```python
from build123d import *

# Parameters (mm, degrees)
SKETCH5_W                                         = 129.54
SKETCH5_H                                         = 88.9
BUTTON_SUPPORT_DEPTH                              = 48.768
SKETCH6_W                                         = 111.76
SKETCH6_H                                         = 60.96
SKETCH6_W_2                                       = 101.6
SKETCH6_H_2                                       = 50.8
BOSS_EXTRUDE4_DEPTH                               = 6.35
SKETCH7_W                                         = 82.55
SKETCH7_H                                         = 50.8
FORCE_SENSOR_CUTOUT_DEPTH                         = 3.81
SKETCH4_W                                         = 129.54
SKETCH4_H                                         = 40.64
BOTTOM_CUT_DEPTH                                  = 139.7
SKETCH25_W                                        = 111.76
SKETCH25_H                                        = 13.97
NEOPIXEL_LIFT_DEPTH                               = 1.778
SKETCH8_W                                         = 5.08
SKETCH8_H                                         = 6.35
HAPTIC_WIRE_HOLES_DEPTH                           = 4.318
SKETCH9_W                                         = 12.7
SKETCH9_H                                         = 12.7
FORCE_SENSOR_HOLE_DEPTH                           = 4.318
SKETCH10_R                                        = 1.0795
NEOPIXEL_HOLES_DEPTH                              = 9.906
NEOPIXEL_WIRE_SIDE_HOLES_REACH                    = 10.128
SKETCH18_W                                        = 8.89
SKETCH18_H                                        = 60.96
SKETCH19_W                                        = 12.7
SKETCH19_H                                        = 13.97
SKETCH19_W_2                                      = 17.78
NEOPIXEL_SOLDER_GAP_DEPTH                         = 5.08
BOSS_EXTRUDE6_DEPTH                               = 1.27
SKETCH11_W                                        = 88.9
SKETCH11_H                                        = 8.128
BOSS_EXTRUDE5_DEPTH                               = 10.16
CSK_FOR_8_FLAT_HEAD_MACHINE_SCREW_100_D           = 4.4958
CSK_FOR_8_FLAT_HEAD_MACHINE_SCREW_100_CSINK_D     = 8.4328
CSK_FOR_8_FLAT_HEAD_MACHINE_SCREW_100_CSINK_ANGLE = 100
SKETCH23_W                                        = 12.7
SKETCH23_H                                        = 13.97
SKETCH23_H_2                                      = 15.24
CUT_EXTRUDE1_DEPTH                                = 5.826
SKETCH24_W                                        = 6.858
SKETCH24_H                                        = 6.35
CUT_EXTRUDE2_DEPTH                                = 121.65


with BuildPart() as part:
    # Sketch5 → Button Support (new body)
    with BuildSketch(Plane(origin=(0, 5.08, 0), x_dir=(1, 0, 0), z_dir=(0, 1, 0))):
        with Locations((69.85, 60.96)):
            Rectangle(SKETCH5_W, SKETCH5_H)
    extrude(amount=BUTTON_SUPPORT_DEPTH)

    # Sketch6 → Boss-Extrude4 (add)
    with BuildSketch(Plane(origin=(0, 53.848, 0), x_dir=(1, 0, 0), z_dir=(0, 1, 0))):
        with Locations((69.85, 60.96)):
            Rectangle(SKETCH6_W, SKETCH6_H)
        with Locations((69.85, 60.96)):
            Rectangle(SKETCH6_W_2, SKETCH6_H_2, mode=Mode.SUBTRACT)
    extrude(amount=BOSS_EXTRUDE4_DEPTH)

    # Sketch7 → Force Sensor Cutout (cut)
    with BuildSketch(Plane(origin=(0, 53.848, 0), x_dir=(1, 0, 0), z_dir=(0, 1, 0))):
        with Locations((69.85, 60.96)):
            Rectangle(SKETCH7_W, SKETCH7_H)
    extrude(amount=-FORCE_SENSOR_CUTOUT_DEPTH, mode=Mode.SUBTRACT)

    # Sketch4 → Bottom Cut (cut)
    with BuildSketch(Plane.XY):
        with Locations((69.85, 25.4)):
            Rectangle(SKETCH4_W, SKETCH4_H)
    extrude(amount=-BOTTOM_CUT_DEPTH, mode=Mode.SUBTRACT)

    # Sketch25 → NeoPixel Lift (add)
    with BuildSketch(Plane(origin=(0, 53.848, 0), x_dir=(1, 0, 0), z_dir=(0, 1, 0))):
        with Locations((69.85, 98.425)):
            Rectangle(SKETCH25_W, SKETCH25_H)
        with Locations((69.85, 23.495)):
            Rectangle(SKETCH25_W, SKETCH25_H)
    extrude(amount=NEOPIXEL_LIFT_DEPTH)

    # Sketch8 → Haptic Wire Holes (cut)
    with BuildSketch(Plane(origin=(0, 50.038, 0), x_dir=(1, 0, 0), z_dir=(0, 1, 0))):
        with Locations((72.898, 67.528002358)):
            Rectangle(SKETCH8_W, SKETCH8_H)
        with Locations((98.298, 67.528002358)):
            Rectangle(SKETCH8_W, SKETCH8_H)
        with Locations((47.498, 67.528002358)):
            Rectangle(SKETCH8_W, SKETCH8_H)
    extrude(amount=-HAPTIC_WIRE_HOLES_DEPTH, mode=Mode.SUBTRACT)

    # Sketch9 → Force Sensor Hole (cut)
    with BuildSketch(Plane(origin=(0, 50.038, 0), x_dir=(1, 0, 0), z_dir=(0, 1, 0))):
        with Locations((46.355, 57.15)):
            Rectangle(SKETCH9_W, SKETCH9_H)
    extrude(amount=-FORCE_SENSOR_HOLE_DEPTH, mode=Mode.SUBTRACT)

    # Sketch10 → NeoPixel Holes (cut)
    with BuildSketch(Plane(origin=(0, 55.626, 0), x_dir=(1, 0, 0), z_dir=(0, 1, 0))):
        with Locations((108.018583302, 19.2294764)):
            Circle(SKETCH10_R)
        with Locations((82.42609372, 19.2294764)):
            Circle(SKETCH10_R)
        with Locations((56.918583394, 19.2294764)):
            Circle(SKETCH10_R)
        with Locations((31.326093812, 19.2294764)):
            Circle(SKETCH10_R)
        with Locations((31.326093812, 102.6905236)):
            Circle(SKETCH10_R)
        with Locations((56.918583394, 102.6905236)):
            Circle(SKETCH10_R)
        with Locations((82.42609372, 102.6905236)):
            Circle(SKETCH10_R)
        with Locations((108.018583302, 102.6905236)):
            Circle(SKETCH10_R)
    extrude(amount=-NEOPIXEL_HOLES_DEPTH, mode=Mode.SUBTRACT)

    # Sketch18 → Neopixel Wire Side Holes (cut, up to next)
    with BuildSketch(Plane(origin=(0, 53.848, 0), x_dir=(1, 0, 0), z_dir=(0, 1, 0)), mode=Mode.PRIVATE) as neopixel_wire_side_holes_sk1:
        with Locations((130.175, 60.96)):
            Rectangle(SKETCH18_W, SKETCH18_H)
    neopixel_wire_side_holes_tool1 = extrude(neopixel_wire_side_holes_sk1.sketch, amount=-NEOPIXEL_WIRE_SIDE_HOLES_REACH, mode=Mode.PRIVATE) & part.part
    add(neopixel_wire_side_holes_tool1.solids().sort_by_distance((130.175, 53.848, -60.96))[0], mode=Mode.SUBTRACT)
    # Sketch18 → Neopixel Wire Side Holes (cut, up to next)
    with BuildSketch(Plane(origin=(0, 53.848, 0), x_dir=(1, 0, 0), z_dir=(0, 1, 0)), mode=Mode.PRIVATE) as neopixel_wire_side_holes_sk2:
        with Locations((9.525, 60.96)):
            Rectangle(SKETCH18_W, SKETCH18_H)
    neopixel_wire_side_holes_tool2 = extrude(neopixel_wire_side_holes_sk2.sketch, amount=-NEOPIXEL_WIRE_SIDE_HOLES_REACH, mode=Mode.PRIVATE) & part.part
    add(neopixel_wire_side_holes_tool2.solids().sort_by_distance((9.525, 53.848, -60.96))[0], mode=Mode.SUBTRACT)

    # Sketch19 → NeoPixel solder gap (cut)
    with BuildSketch(Plane(origin=(0, 55.626, 0), x_dir=(1, 0, 0), z_dir=(0, 1, 0))):
        with Locations((69.85, 98.425)):
            Rectangle(SKETCH19_W, SKETCH19_H)
        with Locations((13.97, 98.425)):
            Rectangle(SKETCH19_W_2, SKETCH19_H)
        with Locations((125.73, 98.425)):
            Rectangle(SKETCH19_W_2, SKETCH19_H)
    neopixel_solder_gap = extrude(amount=-NEOPIXEL_SOLDER_GAP_DEPTH, mode=Mode.SUBTRACT)

    # Mirror1: NeoPixel solder gap across plane
    add(neopixel_solder_gap.mirror(Plane.XY.offset(-60.96)), mode=Mode.SUBTRACT)

    # Sketch20 → Boss-Extrude6 (add)
    with BuildSketch(Plane.XY.offset(-16.51)):
        Polygon((22.86, 50.546), (5.08, 50.546), (5.08, 45.786808958), (134.62, 45.786808958), (134.62, 50.546), (116.84, 50.546), (116.84, 53.848), (76.2, 53.848), (76.2, 50.546), (63.5, 50.546), (63.5, 53.848), (22.86, 53.848), align=None)
    extrude(amount=BOSS_EXTRUDE6_DEPTH)

    # Sketch11 → Boss-Extrude5 (add)
    with BuildSketch(Plane.XY.offset(-15.24)):
        with Locations((69.85, 49.784)):
            Rectangle(SKETCH11_W, SKETCH11_H)
    extrude(amount=BOSS_EXTRUDE5_DEPTH)

    # CSK for #8 Flat Head Machine Screw (100)1 (through all)
    with Locations(Plane(origin=(0, 50.546, 0), x_dir=(1, 0, 0), z_dir=(0, 1, 0))):
        with Locations((12.7, 99.06), (127, 99.06), (127, 21.59), (12.7, 21.59)):
            CounterSinkHole(CSK_FOR_8_FLAT_HEAD_MACHINE_SCREW_100_D / 2, CSK_FOR_8_FLAT_HEAD_MACHINE_SCREW_100_CSINK_D / 2, counter_sink_angle=CSK_FOR_8_FLAT_HEAD_MACHINE_SCREW_100_CSINK_ANGLE)

    # Sketch23 → Cut-Extrude1 (cut, through all)
    with BuildSketch(Plane(origin=(0, 50.546, 0), x_dir=(1, 0, 0), z_dir=(0, 1, 0))):
        with Locations((69.85, 98.425)):
            Rectangle(SKETCH23_W, SKETCH23_H)
        with Locations((69.85, 22.86)):
            Rectangle(SKETCH23_W, SKETCH23_H_2)
    extrude(amount=-CUT_EXTRUDE1_DEPTH, mode=Mode.SUBTRACT)

    # Sketch24 → Cut-Extrude2 (cut, through all)
    with BuildSketch(Plane(origin=(125.73, 0, 0), x_dir=(0, 0, -1), z_dir=(1, 0, 0))):
        with Locations((69.215, 57.023)):
            Rectangle(SKETCH24_W, SKETCH24_H)
    extrude(amount=-CUT_EXTRUDE2_DEPTH, mode=Mode.SUBTRACT)


solid = part.part
```
The listing builds one solid part. Answer for the finished solid, in the listing's coordinates (mm). A direction names the side the tool comes from. Round coordinates to 2 decimals unless told otherwise and drop trailing zeros. Loops run counter-clockwise (first coordinate to the right, second up) from the corner with the lowest first, then second, coordinate; pieces in that order, holes last.
Q1. Given pin 1 Ø7 at (y, z) = (57.5, -56) entering from +X; pin 2 Ø0.9 at (x, y) = (40, 54.5) entering from +Z; pin 3 Ø7 at (x, z) = (18, -96.5) entering from +Y, each flat-ended and moving along its own axis, determine where each tip first touches the part or whether it passes through.
Q2. Section C-C, the plane z = -45.5 is taken. Determine the outline of the cut face in (x, y) (3 decimals), then the cut area to 3 significant figures.
Q3. Section A-A, the plane z = -99.06 is taken. Determine the outline of the cut face in (x, y), then the cut area to 3 significant figures.
Q4. Section D-D, the plane x = 88.5 is taken. Determine the outline of the cut face in (y, z).
Q5. For a pull along Z with two mould halves and no side action, classify faces 1 (the face through (17, 57, -72.644)), 2 (the face through (124, 50.546, -95)), 3 (the face through (69, 56, -30.48)) as released by +Z, released by -Z, zero draft, split by the parting line, or undercut.
Q6. Section B-B, the plane x = 67 is taken. Determine the outline of the cut face in (y, z).
Q7. Which of the six approach directions +Z, -Z, +X, -X, +Y, -Y give full straight-line access (tool end or side, diameter ignored) to faces 4 (the face through (120.65, 57, -50)), 5 (the face through (22.86, 53, -23)), 6 (the face through (25.4, 50, -10)), 7 (the face through (123, 57, -65.786)), 8 (the face through (95.758, 48, -67))?
Q8. Find the intervals of material crossed by line 1 (Z direction, x = 127, y = 47.35); line 2 (X direction, y = 46.95, z = -21.59); line 3 (Z direction, x = 26, y = 57.75), in increasing order.
Completed:
1. pin 1: stops at x = 125.73
1. pin 2: stops at z = -16.51
1. pin 3: stops at y = 50.55
2. outline: (13.97, 45.72) - (125.73, 45.72) - (125.73, 60.198) - (120.65, 60.198) - (120.65, 53.848) - (111.125, 53.848) - (111.125, 50.038) - (28.575, 50.038) - (28.575, 53.848) - (19.05, 53.848) - (19.05, 60.198) - (13.97, 60.198) - close
2. area: 658 mm2
3. outline: (5.08, 45.72) - (10.45, 45.72) - (10.45, 48.89) - (8.48, 50.55) - (5.08, 50.55) - close; (14.95, 45.72) - (63.5, 45.72) - (63.5, 55.63) - (22.86, 55.63) - (22.86, 50.55) - (16.92, 50.55) - (14.95, 48.89) - close; (76.2, 45.72) - (124.75, 45.72) - (124.75, 48.89) - (122.78, 50.55) - (116.84, 50.55) - (116.84, 55.63) - (76.2, 55.63) - close; (129.25, 45.72) - (134.62, 45.72) - (134.62, 50.55) - (131.22, 50.55) - (129.25, 48.89) - close
3. area: 927 mm2
4. outline: (45.72, -105.41) - (55.63, -105.41) - (55.63, -91.44) - (60.2, -91.44) - (60.2, -86.36) - (50.04, -86.36) - (50.04, -35.56) - (60.2, -35.56) - (60.2, -30.48) - (55.63, -30.48) - (55.63, -16.51) - (53.85, -16.51) - (53.85, -5.08) - (45.72, -5.08) - (45.72, -15.24) - (45.79, -15.24) - (45.79, -16.51) - (45.72, -16.51) - close
5. face 1: undercut
5. face 2: zero draft
5. face 3: undercut
6. outline: (45.72, -91.44) - (60.2, -91.44) - (60.2, -86.36) - (50.04, -86.36) - (50.04, -35.56) - (60.2, -35.56) - (60.2, -30.48) - (45.72, -30.48) - close; (45.72, -15.24) - (53.85, -15.24) - (53.85, -5.08) - (45.72, -5.08) - close
7. face 4: +Y
7. face 5: +Z, -X, +Y
7. face 6: +Z, -X, +Y, -Y
7. face 7: +X, -X, +Y
7. face 8: +Y, -Y
8. line 1: z = -105.41 to -101.31, -96.81 to -91.44, -30.48 to -23.84, -19.34 to -15.24
8. line 2: x = 5.08 to 10.45, 14.95 to 63.5, 76.2 to 124.75, 129.25 to 134.62
8. line 3: z = -91.44 to -86.36, -35.56 to -30.48
